Autodesk Inventor part; units mm, degrees
ref_plane "YZ Plane" through (0, 0, 0) normal (1, 0, 0) x (0, 1, 0)
ref_plane "XZ Plane" through (0, 0, 0) normal (0, 1, 0) x (-1, 0, 0)
ref_plane "XY Plane" through (0, 0, 0) normal (0, 0, 1) x (1, 0, 0)
sketch "Sketch1" plane through (0, 0, 0) normal (0, 0, 1) x (1, 0, 0)
  line L0 (0, 0) -> (60.325, 0)
  line L1 (60.325, 0) -> (60.325, 38.1)
  line L2 (60.325, 38.1) -> (0, 38.1)
  line L3 (0, 38.1) -> (0, 0)
  dimension "d0" = 60.325
  dimension "d1" = 38.1
extrude "Extrusion1" add sketch "Sketch1" along normal blind 3.429
sketch "Sketch4" plane through (0, 0, 3.429) normal (0, 0, 1) x (1, 0, 0)
  line L0 (60.325, 38.1) -> (0, 38.1)
  line L1 (0, 38.1) -> (0, 0)
  point P0 (30.1625, 19.05)
  point P1 (30.1625, 38.1)
  point P2 (0, 19.05)
hole "Hole1" at (30.1625, 19.05, 3.429) direction (0, 0, -1) diameter 28.575 end through all
sketch "Sketch5" plane through (0, 0, 3.429) normal (0, 0, 1) x (1, 0, 0)
  line L0 (0, 38.1) -> (0, 0)
  point P0 (60.325, 0)
  point P1 (60.325, 38.1)
  point P2 (4.7752, 19.05)
  point P3 (55.5498, 19.05)
  point P4 (0, 19.05)
  point P5 (0, 19.05)
  dimension "d19" = 4.7752
  dimension "d20" = 4.7752
  dimension "d21" = 19.05
  dimension "d22" = 19.05
hole "Hole2" at (4.7752, 19.05, 3.429) at (55.5498, 19.05, 3.429) direction (0, 0, -1) diameter 5.1054 end through all
sketch "Sketch6" plane through (0, 0, 3.429) normal (0, 0, 1) x (1, 0, 0)
  circle A0 centre (30.1625, 19.05) radius 14.2875
  circle A1 centre (30.1625, 19.05) radius 15.875
  dimension "d30" = 31.75
extrude "Extrusion2" cut sketch "Sketch6" against normal blind 1.5875
properties part number "Bearing Reciver for 1-2 bearing"
The listing builds one solid part. Answer for the finished solid, in the listing's coordinates (mm). A direction names the side the tool comes from. Give positions to 0.01 mm unless a question says otherwise; leave off trailing zeros. Order: outer loops, then holes, each group sorted by start corner. A loop starts at its lowest first (then second) coordinate and runs counter-clockwise, first axis right, second up. Notation, with made-up numbers: (68, -21.75) - (82, -21.75) arc R31 ccw to (82, 4.25) - close; hole circle Ø10 at (89.25, -27). An arc over 180 degrees is marked (long way). One line per item, written item: value. Start each with the question number.
1) A cutting plane is placed at C-C on y = 11. Give the vertices of the cut face in (x, z) (1 decimal), then the cut area to 3 significant figures.
2) A tool of negligible diameter and unlimited length cuts with its end or side. For faces 1 (the face through (16, 24, 0)), 2 (the face through (26.721, 3.553, 2.646)), from which of +Z, -Z, +X, -X, +Y, -Y can it reach the whole face along a straight path? Write none if from no direction.
3) A cutting plane is placed at B-B on y = 19.05. State how many separate pieces and enclosed holes the cut face has, then the cut area to 3 significant figures.
4) Find the intervals of material crossed by L1, parallel to X at y = 17, z = 2.35 (3 decimals); L2, parallel to Y at x = 33, z = 0.75; L3, parallel to Y at x = 7, z = 0.55, in increasing order.
5) A cutting plane is placed at A-A on x = 28.5. Give the vertices of the cut face in (y, z), then the cut area to 3 significant figures.
6) The mould has two halves that part along Y. Classify faces 3 (the face through (4.008, 16.615, 1.69)), 4 (the face through (16, 28, 3.429)), 5 (the face through (31, 38.1, 2)), 6 (the face through (17, 25, 1.842)): released by +Y, released by -Y, zero draft, split by the parting line, or undercut.
7) Given pin 1 Ø4 at (x, y) = (4.78, 19.05) entering from +Z, flat-ended and moving along its own axis, determine where the tip first touches the part or whether it passes through.
Answer sheet:
1. outline: (0, 0) - (18.4, 0) - (18.4, 1.8) - (16.5, 1.8) - (16.5, 3.4) - (0, 3.4) - close; (42, 0) - (60.3, 0) - (60.3, 3.4) - (43.8, 3.4) - (43.8, 1.8) - (42, 1.8) - close
1. area: 120 mm2
2. face 1: -Z, +X, -X, +Y, -Y
2. face 2: +Z
3. separate pieces: 4
3. enclosed holes: 0
3. area: 68.8 mm2
4. L1: x = 0 to 3.254, 6.296 to 14.42, 45.905 to 54.029, 57.071 to 60.325
4. L2: y = 0 to 5.05, 33.05 to 38.1
4. L3: y = 0 to 17.8, 20.3 to 38.1
5. outline: (0, 0) - (4.86, 0) - (4.86, 1.84) - (3.26, 1.84) - (3.26, 3.43) - (0, 3.43) - close; (33.24, 0) - (38.1, 0) - (38.1, 3.43) - (34.84, 3.43) - (34.84, 1.84) - (33.24, 1.84) - close
5. area: 28.3 mm2
6. face 3: undercut
6. face 4: zero draft
6. face 5: released by +Y
6. face 6: undercut
7. pin 1: passes through
